Design review of the part built by this model. Coordinates are the model's own, in mm. A direction names the side the tool comes from. Give positions to 0.01 mm unless a question says otherwise; leave off trailing zeros. Order: outer loops, then holes, each group sorted by start corner. A loop starts at its lowest first (then second) coordinate and runs counter-clockwise, first axis right, second up. Notation, with made-up numbers: M -9.75,-32 L 43.25,-32 A20 ccw 43.25,-8 Z; hole C 4.25,2 d4. An arc over 180 degrees is marked long. Put each result on its own line as item: value. Start each with the question number.
Autodesk Inventor part; units mm, degrees
ref_plane "YZ Plane" through (0, 0, 0) normal (1, 0, 0) x (0, 1, 0)
ref_plane "XZ Plane" through (0, 0, 0) normal (0, 1, 0) x (-1, 0, 0)
ref_plane "XY Plane" through (0, 0, 0) normal (0, 0, 1) x (1, 0, 0)
sketch "Schizzo1" plane through (0, 0, 0) normal (0, 0, 1) x (1, 0, 0)
  line L0 (-40, 15) -> (40, 15)
  line L1 (40, 15) -> (40, -15)
  line L2 (40, -15) -> (-40, -15)
  line L3 (-40, -15) -> (-40, 15)
  line L4 (-40, 15) -> (40, -15) construction
  line L5 (40, 15) -> (-40, -15) construction
  point P0 (0, 0)
  dimension "d0" = 80
  dimension "d1" = 30
extrude "Piano1" add sketch "Schizzo1" along normal blind 1.5
sketch "Schizzo2" plane through (40, -14.25, 1.299) normal (0, -0.5, -0.8660254) x (1, 0, 0)
  line L0 (-80, 0) -> (0, 0)
  line L1 (0, 0) -> (0, 30)
  line L2 (0, 30) -> (-80, 30)
  line L3 (-80, 30) -> (-80, 0)
edge flange "Flangia1" height 30 angle 30 thickness 1.5 bend radius 1.5 thickness toward (0, -0.5, -0.8660254) relief tear relief width 1.5 relief depth 0.75 edges at (0, -15, 1.5) wall of the first edge with corners at (-40, -14.25, 1.299) (40, -14.25, 1.299) (40, -40.2308, 16.299) (-40, -40.2308, 16.299)
bend "Piega (Bend)1"
corner "Angolo1"
sketch "Schizzo3" plane through (-40, 14.25, 1.299) normal (0, 0.5, -0.8660254) x (-1, 0, 0)
  line L0 (-80, 0) -> (0, 0)
  line L1 (0, 0) -> (0, 20)
  line L2 (0, 20) -> (-80, 20)
  line L3 (-80, 20) -> (-80, 0)
edge flange "Flangia2" height 20 angle 30 thickness 1.5 bend radius 1.5 thickness toward (0, 0.5, -0.8660254) relief tear relief width 1.5 relief depth 0.75 edges at (0, 15, 1.5) wall of the first edge with corners at (40, 14.25, 1.299) (-40, 14.25, 1.299) (-40, 31.5705, 11.299) (40, 31.5705, 11.299)
bend "Piega (Bend)2"
corner "Angolo2"
sketch "Schizzo4" plane through (-40, -43.0298, 12.951) normal (0, -0.8660254, -0.5) x (1, 0, 0)
  line L0 (80, 0) -> (0, 0)
  line L1 (0, 0) -> (0, -23.8038)
  line L2 (0, -23.8038) -> (80, -23.8038)
  line L3 (80, -23.8038) -> (80, 0)
edge flange "Flangia3" height 35 angle 150 thickness 1.5 bend radius 1.5 thickness toward (0, -0.8660254, -0.5) relief tear relief width 1.5 relief depth 0.75 edges at (0, -40.9808, 15) wall of the first edge with corners at (40, -43.0298, 12.951) (-40, -43.0298, 12.951) (-40, -31.1279, -7.6638) (40, -31.1279, -7.6638)
bend "Piega (Bend)3"
corner "Angolo3"
sketch "Schizzo6" plane through (-40, -30.1663, -8.3753) normal (0, -0.2249511, -0.9743701) x (1, 0, 0)
  line L0 (80, 0) -> (0, 0)
  line L1 (0, 0) -> (0, -28.6956)
  line L2 (0, -28.6956) -> (80, -28.6956)
  line L3 (80, -28.6956) -> (80, 0)
edge flange "Flangia5" height 30 angle 47 thickness 1.5 bend radius 1.5 thickness toward (0, -0.2249511, -0.9743701) relief tear relief width 1.5 relief depth 0.75 edges at (0, -31.1279, -7.6638) wall of the first edge with corners at (40, -30.1663, -8.3753) (-40, -30.1663, -8.3753) (-40, -2.2062, -14.8304) (40, -2.2062, -14.8304)
bend "Piega (Bend)5"
corner "Angolo5"
sketch "Schizzo7" plane through (40, -2.5436, -16.292) normal (0, -0.2249511, -0.9743701) x (-1, 0, 0)
  line L0 (80, 0) -> (80, -28.6956)
  line L1 (0, 0) -> (80, 0)
  point P0 (40, -1.1865)
  point P1 (40, -14.3478)
  point P2 (80, -14.3478)
  point P3 (40, 0)
hole "Foro1" at (0, -16.5236, -13.0644) direction (0, 0.2249511, 0.9743701) diameter 10 depth 1.5 tip angle 118
fillet "Arrotondamento angolo1" radius 10 4 edges at (-40, 31.9455, 10.6495) (40, 31.9455, 10.6495) (40, -2.3749, -15.5612) (-40, -2.3749, -15.5612)
equation "\"d58\" = Spessore"
equation "\"d2\" = Spessore"
equation "\"d3\" = LarghezzaScaricoPiega"
equation "\"d4\" = ProfonditàScaricoPiega"
equation "\"d5\" = ResiduoMinimo"
equation "\"d6\" = RaggioTransizione"
equation "\"d9\" = RaggioPiega"
equation "\"d10\" = DimensioniScaricoAngolo"
equation "\"d11\" = DimensioneGioco"
equation "\"d12\" = Dimensione_raggio_Jacobi"
equation "\"d13\" = LarghezzaScaricoPiega"
equation "\"d14\" = ProfonditàScaricoPiega"
equation "\"d15\" = ResiduoMinimo"
equation "\"d16\" = RaggioTransizione"
equation "\"d19\" = RaggioPiega"
equation "\"d20\" = DimensioniScaricoAngolo"
equation "\"d21\" = DimensioneGioco"
equation "\"d22\" = Dimensione_raggio_Jacobi"
equation "\"d23\" = LarghezzaScaricoPiega"
equation "\"d24\" = ProfonditàScaricoPiega"
equation "\"d25\" = ResiduoMinimo"
equation "\"d26\" = RaggioTransizione"
equation "\"d29\" = RaggioPiega"
equation "\"d30\" = DimensioniScaricoAngolo"
equation "\"d31\" = DimensioneGioco"
equation "\"d32\" = Dimensione_raggio_Jacobi"
equation "\"d43\" = LarghezzaScaricoPiega"
equation "\"d44\" = ProfonditàScaricoPiega"
equation "\"d45\" = ResiduoMinimo"
equation "\"d46\" = RaggioTransizione"
equation "\"d49\" = RaggioPiega"
equation "\"d50\" = DimensioniScaricoAngolo"
equation "\"d51\" = DimensioneGioco"
equation "\"d52\" = Dimensione_raggio_Jacobi"
equation "\"RaggioPiega\" = Spessore"
equation "\"LarghezzaScaricoPiega\" = Spessore"
equation "\"ProfonditàScaricoPiega\" = 0.5 * Spessore"
equation "\"DimensioniScaricoAngolo\" = 4 * Spessore"
equation "\"ResiduoMinimo\" = 2 * Spessore"
equation "\"RaggioTransizione\" = RaggioPiega"
equation "\"Dimensione_raggio_Jacobi\" = RaggioPiega"
equation "\"DimensioneGioco\" = Spessore"
properties part number "Lamiera pinza"
1. Consider section A-A on x = -22. Give the boundary of the cut face in (y, z).
2. The part is to be moulded in two halves that separate along X. For faces 6 (the cylindrical face through (-0.22, -21.22, -11.2)), 7 (the cylindrical face through (-37.148, 29.347, 9.137)), 8 (the cylindrical face through (36.993, 29.481, 9.215)), 9 (the flat face through (-1, 0, 1.5)), say which applies: +X half, -X half, draft (parallel to the pull), parting line (faces both ways), or undercut.
3. Insertion check: pin 1 (5 mm diameter, centred on x = 21.5, y = 11.5, fed in from -Z); pin 2 (1.5 mm diameter, centred on x = 21, z = -3.5, fed in from -Y); pin 3 (12 mm diameter, centred on x = 15.5, y = -25.5, fed in from -Z). Each pin has a flat end and moves straight along its axis. Give the tip position at first contact, or say it passes through.
4. Consider section C-C on z = 14. Give the boundary of the cut face in (x, y).
5. To check wall thickness, follow probe 1 along Y at (x, z) = (-1, 7); probe 2 along Y at (x, z) = (-18, 3); probe 3 along Z at (x, y) = (3, 4.5). State the ranges of each line that lie inside material, in increasing order.
6. Consider section B-B on y = -34. Give the boundary of the cut face in (x, z), then the cut area to 3 significant figures.
7. Consider section D-D on y = 3.5. Give the boundary of the cut face in (x, z).
8. Machinability: for faces 1 (the flat face through (-0.56, -22.595, -10.123)), 2 (the flat face through (0.56, -27.412, 8.898)), 3 (the flat face through (0.56, -28.516, 7.803)), 4 (the flat face through (40, -18, 2)), 5 (the cylindrical face through (-37.15, -5.31, -14.89)), which of the approach directions +Z, -Z, +X, -X, +Y, -Y give a long, thin tool a straight path to every point of the face, cutting with its end or side? Answer none if there is none.
Returned:
1. outline: M -44.33,12.2 L -32.43,-8.41 A3 ccw -30.5,-9.84 L -2.54,-16.29 L -2.21,-14.83 L -30.17,-8.38 A1.5 cw -31.13,-7.66 L -43.03,12.95 A1.5 cw -40.98,15 L -15.7,0.4 A3 ccw -14.2,0 L 14.2,0 A3 ccw 15.7,0.4 L 32.32,10 L 31.57,11.3 L 14.95,1.7 A1.5 cw 14.2,1.5 L -14.2,1.5 A1.5 cw -14.95,1.7 L -40.23,16.3 A3 ccw Z
2. face 6: undercut
2. face 7: -X half
2. face 8: +X half
2. face 9: draft
3. pin 1: stops at z = 0
3. pin 2: stops at y = -35.7
3. pin 3: stops at z = -12.38
4. outline: M -40,-44.72 L 40,-44.72 L 40,-43.2 L -40,-43.2 Z; M -40,-39.25 L 40,-39.25 L 40,-36.25 L -40,-36.25 Z
5. probe 1: y = -41.33 to -39.59, -27.12 to -24.12, 24.12 to 27.12
5. probe 2: y = -39.02 to -37.28, -20.2 to -17.2, 17.2 to 20.2
5. probe 3: z = 0 to 1.5
6. outline: M -40,-5.69 L 40,-5.69 L 40,-2.69 L -40,-2.69 Z; M -40,10.97 L 40,10.97 L 40,12.7 L -40,12.7 Z
6. area: 379 mm2
7. outline: M -40,0 L 40,0 L 40,1.5 L -40,1.5 Z
8. face 1: +X, -X, +Y
8. face 2: +Z, +X, -X
8. face 3: +X, -X
8. face 4: +Z, -Z, +X, +Y, -Y
8. face 5: -Z, -X, +Y
